from build123d import *

# Parameters (mm, degrees)
BOSS_EXTRUDE1_DEPTH  = 6
SKETCH2_W            = 6
SKETCH2_H            = 5
BOSS_EXTRUDE2_DEPTH  = 20
EXTRUDE_1_DEPTH      = 15
EXTRUDE_1_DEPTH_BACK = 10.2
SKETCH_2_W           = 6
SKETCH_2_H           = 2
FILLET_3_R           = 1


with BuildPart() as part:
    # Sketch1 → Boss-Extrude1 (new body)
    with BuildSketch(Plane.XY):
        with BuildLine():
            Line((-3.6, 0), (-3.6, 17))
            ThreePointArc((-3.6, 17), (0, 20.6), (3.6, 17))
            Line((3.6, 17), (3.6, 0))
            Line((3.6, 0), (3.6, -10.95432829))
            Line((3.6, -10.95432829), (-3.6, -10.95432829))
            Line((-3.6, -10.95432829), (-3.6, 0))
        make_face()
        with BuildLine():
            Line((-0.6, 0), (-0.6, 17))
            ThreePointArc((-0.6, 17), (0, 17.6), (0.6, 17))
            Line((0.6, 17), (0.6, 0))
            ThreePointArc((0.6, 0), (0, -0.6), (-0.6, 0))
        make_face(mode=Mode.SUBTRACT)
    extrude(amount=BOSS_EXTRUDE1_DEPTH)

    # Sketch2 → Boss-Extrude2 (add)
    with BuildSketch(Plane(origin=(3.6, 0, 0), x_dir=(0, 0, -1), z_dir=(1, 0, 0))):
        with Locations((-3, 3.022835855)):
            Rectangle(SKETCH2_W, SKETCH2_H)
    extrude(amount=BOSS_EXTRUDE2_DEPTH)

    # Эскиз2 → Бобышка-Вытянуть1 (add, two sides: drawn at the far end of the back side and taken through both)
    with BuildSketch(Plane(origin=(3.6, 0, 0), x_dir=(0, 0, -1), z_dir=(1, 0, 0)).offset(-EXTRUDE_1_DEPTH_BACK)):
        with Locations((-3, -9.95432829)):
            Rectangle(SKETCH_2_W, SKETCH_2_H)
    extrude(amount=EXTRUDE_1_DEPTH + EXTRUDE_1_DEPTH_BACK)

    # Скругление3
    fillet_3_edges = [part.edges().sort_by_distance(p)[0] for p in [
        (-6.6, -10.95432829, 3),
        (18.6, -10.95432829, 3),
    ]]
    fillet(fillet_3_edges, radius=FILLET_3_R)


solid = part.part
Can you work these out from the model? Positions are in its coordinate system, mm. A direction names the side the tool comes from. Coordinates: 2 decimals unless noted, no trailing zeros. Order: outer loops, then holes, each group sorted by start corner. A loop starts at its lowest first (then second) coordinate and runs counter-clockwise, first axis right, second up. Notation, with made-up numbers: M 41,15 L 59,15 A18 ccw 59,31 Z; hole C 87.25,20.25 d11. An arc over 180 degrees is marked long. Write item = value, one per line.
(1) Suppose I cut it at C-C on z = 4.8. Please give me the cut outline in (x, y).
Results are:
outline = M -6.6,-9.95 A1 ccw -5.6,-10.95 L 17.6,-10.95 A1 ccw 18.6,-9.95 L 18.6,-8.95 L 3.6,-8.95 L 3.6,0.52 L 23.6,0.52 L 23.6,5.52 L 3.6,5.52 L 3.6,17 A3.6 ccw -3.6,17 L -3.6,-8.95 L -6.6,-8.95 Z; hole M -0.6,0 A0.6 ccw 0.6,0 L 0.6,17 A0.6 ccw -0.6,17 Z
(2) For faces 4 (the face through (-3.6, 4, 3)), 5 (the face through (-0.6, 8, 3)), 6 (the face through (13, 5.523, 3)), 7 (the face through (11, -8.954, 3)), which set-ups out of +Z, -Z, +X, -X, +Y, -Y let a thin tool reach every point of the face, with its end or its side?
Results are:
face_4 = +Z, -Z, -X, +Y
face_5 = +Z, -Z
face_6 = +Z, -Z, +X, +Y
face_7 = +Z, -Z, +X
(3) Suppose I cut it at D-D on y = -5. Please give me the cut outline in (x, z), plus the area to 3 significant figures.
Results are:
outline = M -3.6,0 L 3.6,0 L 3.6,6 L -3.6,6 Z
area = 43.2 mm2
(4) Suppose I cut it at A-A on x = 0. Please give me the cut outline in (y, z).
Results are:
outline = M -10.95,0 L -0.6,0 L -0.6,6 L -10.95,6 Z; M 17.6,0 L 20.6,0 L 20.6,6 L 17.6,6 Z
(5) I need wall thicknesses on line 1 along Y through (x, z) = (12, 1.45); line 2 along X through (y, z) = (3, 4.4); line 3 along X through (y, z) = (17, 4.75). Which ranges of each line are inside material? Lowest first, please. Write a range as [from, to].
Results are:
line_1 = [-10.95, -8.95], [0.52, 5.52]
line_2 = [-3.6, -0.6], [0.6, 23.6]
line_3 = [-3.6, -0.6], [0.6, 3.6]
(6) For pin 1 Ø1.8 at (y, z) = (11.5, 2.5) entering from +X; pin 2 Ø1.8 at (y, z) = (5, 4) entering from -X; pin 3 Ø0.8 at (y, z) = (-9.5, 4.5) entering from +X, each with a flat end and sliding along its axis, tell me the tip position at first contact or that it passes through.
Results are:
pin_1 = 3.6
pin_2 = -3.6
pin_3 = 18.6
(7) If we mould it in two halves opening along Y, with no side actions, what happens to faces 1 (the face through (13, 0.523, 3)), 2 (the face through (23.6, 3, 3)), 3 (the face through (-5, -8.954, 3))? For each: pulls with the +Y half, pulls with the -Y half, needs draft (parallel to the pull), parting line crosses it, or undercut.
Results are:
face_1 = undercut
face_2 = needs draft
face_3 = pulls with the +Y half
(8) Suppose I cut it at B-B on y = 16. Please give me the cut outline in (x, z).
Results are:
outline = M -3.6,0 L -0.6,0 L -0.6,6 L -3.6,6 Z; M 0.6,0 L 3.6,0 L 3.6,6 L 0.6,6 Z
